from build123d import *

# Parameters (mm, degrees)
F1_DEPTH  = 1120.775
F3_DEPTH  = 53.34
F6_DEPTH  = 565.15
F8_DEPTH  = 55.5625
F10_DEPTH = 45.155127
F12_DEPTH = 25.4
F14_DEPTH = 25.4
F16_DEPTH = 55.5625
F18_DEPTH = 49.193727
F20_DEPTH = 25.4
F22_DEPTH = 113.792
F24_DEPTH = 25.4
F26_DEPTH = 25.4
F28_DEPTH = 25.4
F30_DEPTH = 254
F32_DEPTH = 63.5
F34_DEPTH = 25.4
F36_DEPTH = 25.4
F38_DEPTH = 25.4
F40_DEPTH = 25.4
F41_W     = 53.975
F41_H     = 53.975
F42_DEPTH = 1239.52
F43_R     = 10.31875
F44_DEPTH = 89.662
F45_R     = 10.31875
F46_DEPTH = 179.832


with BuildPart() as f1:
    # F0 (on Front) → F1 (new body)
    with BuildSketch(Plane.XZ):
        Polygon((30.1625, 30.1625), (26.9875, 30.1625), (-26.9875, 30.1625), (-30.1625, 30.1625), (-30.1625, 26.9875), (-30.1625, -26.9875), (-30.1625, -30.1625), (-26.9875, -30.1625), (26.9875, -30.1625), (30.1625, -30.1625), (30.1625, -26.9875), (30.1625, 26.9875), align=None)
        Polygon((-23.8125, 26.9875), (23.8125, 26.9875), (26.9875, 26.9875), (26.9875, 23.8125), (26.9875, -23.8125), (26.9875, -26.9875), (23.8125, -26.9875), (-23.8125, -26.9875), (-26.9875, -26.9875), (-26.9875, -23.8125), (-26.9875, 23.8125), (-26.9875, 26.9875), align=None, mode=Mode.SUBTRACT)
    extrude(amount=-F1_DEPTH)

    # F2 (on Right) → F3 (cut, symmetric)
    with BuildSketch(Plane.YZ):
        Polygon((569.9125, 80.052234), (569.9125, 0), (569.9125, -86.322285), (989.0125, -86.322285), (989.0125, 80.052234), align=None)
    extrude(amount=F3_DEPTH, both=True, mode=Mode.SUBTRACT)



with BuildPart() as f6:
    # F5 (on offset) → F6 (new body)
    with BuildSketch(Plane.XZ.offset(-468.3125)):
        Polygon((-20.5486, 35.0139), (-20.5486, 30.2514), (30.2514, 30.2514), (30.2514, -19.031227), (35.0139, -19.031227), (35.0139, 35.0139), align=None)
        Polygon((-30.2514, 19.031227), (-35.0139, 19.031227), (-35.0139, -35.0139), (20.5486, -35.0139), (20.5486, -30.2514), (-30.2514, -30.2514), align=None)
    extrude(amount=-F6_DEPTH)


with BuildPart() as f1_1:
    add(f1.part)

    add(f6.part)  # F8 merges F6
    # F7 (on face) → F8 (join, through all)
    with BuildSketch(Plane(origin=(-20.5486, 0, 0), x_dir=(0, -1, 0), z_dir=(-1, 0, 0))):
        Polygon((-1033.4625, 30.2514), (-1033.4625, 35.0139), (-1042.3525, 26.1239), (-1033.4625, 26.1239), align=None)
        Polygon((-459.4225, 26.1239), (-468.3125, 35.0139), (-468.3125, 30.2514), (-468.3125, 26.1239), align=None)
    extrude(amount=-F8_DEPTH)

    # F9 (on face) → F10 (join, through all)
    with BuildSketch(Plane(origin=(0, 0, -19.031227), x_dir=(1, 0, 0), z_dir=(0, 0, -1))):
        Polygon((30.2514, -468.3125), (35.0139, -468.3125), (26.1239, -459.4225), (26.1239, -468.3125), align=None)
        Polygon((26.1239, -1042.3525), (35.0139, -1033.4625), (30.2514, -1033.4625), (26.1239, -1033.4625), align=None)
    extrude(amount=-F10_DEPTH)

    # F11 (on face) → F12 (cut)
    with BuildSketch(Plane(origin=(0, 0, 26.1239), x_dir=(1, 0, 0), z_dir=(0, 0, -1))):
        Polygon((35.0139, -459.4225), (30.1625, -459.4225), (30.1625, -463.4611), (35.0139, -468.3125), align=None)
    extrude(amount=-F12_DEPTH, mode=Mode.SUBTRACT)

    # F13 (on face) → F14 (cut)
    with BuildSketch(Plane(origin=(0, 0, 26.1239), x_dir=(1, 0, 0), z_dir=(0, 0, -1))):
        Polygon((35.0139, -1042.3525), (35.0139, -1033.4625), (30.1625, -1038.3139), (30.1625, -1042.3525), align=None)
    extrude(amount=-F14_DEPTH, mode=Mode.SUBTRACT)

    # F15 (on face) → F16 (join, through all)
    with BuildSketch(Plane.YZ.offset(20.5486)):
        Polygon((459.4225, -26.1239), (468.3125, -35.0139), (468.3125, -26.1239), align=None)
        Polygon((1033.4625, -26.1239), (1033.4625, -35.0139), (1042.3525, -26.1239), align=None)
    extrude(amount=-F16_DEPTH)

    # F17 (on face) → F18 (join, through all)
    with BuildSketch(Plane.XY.offset(19.031227)):
        Polygon((-26.1239, 468.3125), (-35.0139, 468.3125), (-26.1239, 459.4225), align=None)
        Polygon((-26.1239, 1042.3525), (-35.0139, 1033.4625), (-26.1239, 1033.4625), align=None)
    extrude(amount=-F18_DEPTH)

    # F19 (on face) → F20 (cut)
    with BuildSketch(Plane.XY.offset(-26.1239)):
        Polygon((-35.0139, 1033.4625), (-30.1625, 1038.3139), (-30.1625, 1042.3525), (-35.0139, 1042.3525), align=None)
    extrude(amount=-F20_DEPTH, mode=Mode.SUBTRACT)

    # F21 (on face) → F22 (join)
    with BuildSketch(Plane(origin=(0, 569.9125, 0), x_dir=(-1, 0, 0), z_dir=(0, 1, 0))):
        Polygon((29.4386, 26.1239), (20.5486, 35.0139), (20.5486, 26.1239), (26.1239, 26.1239), (26.1239, 27.921227), (27.921227, 26.1239), align=None)
        Polygon((27.921227, 26.1239), (26.1239, 26.1239), (26.1239, 19.031227), (35.0139, 19.031227), align=None)
        Polygon((-26.1239, -26.1239), (-26.1239, -19.031227), (-35.0139, -19.031227), (-27.921227, -26.1239), align=None)
        Polygon((-20.5486, -26.1239), (-26.1239, -26.1239), (-26.1239, -27.921227), (-27.921227, -26.1239), (-29.4386, -26.1239), (-20.5486, -35.0139), align=None)
    extrude(amount=-F22_DEPTH)

    # F23 (on face) → F24 (cut)
    with BuildSketch(Plane(origin=(20.5486, 0, 0), x_dir=(0, -1, 0), z_dir=(-1, 0, 0))):
        Polygon((-468.3125, -35.0139), (-456.1205, -35.0139), (-456.1205, -30.1625), (-463.4611, -30.1625), align=None)
    extrude(amount=-F24_DEPTH, mode=Mode.SUBTRACT)

    # F25 (on face) → F26 (cut)
    with BuildSketch(Plane.XY.offset(-19.031227)):
        Polygon((35.0139, 468.3125), (30.1625, 463.4611), (30.1625, 456.1205), (35.0139, 456.1205), align=None)
    extrude(amount=-F26_DEPTH, mode=Mode.SUBTRACT)

    # F27 (on face) → F28 (cut)
    with BuildSketch(Plane.YZ.offset(-20.5486)):
        Polygon((456.1205, 35.0139), (456.1205, 30.1625), (463.4611, 30.1625), (468.3125, 35.0139), align=None)
    extrude(amount=-F28_DEPTH, mode=Mode.SUBTRACT)

    # F29 (on face) → F30 (cut, symmetric)
    with BuildSketch(Plane(origin=(0, 0, 19.031227), x_dir=(1, 0, 0), z_dir=(0, 0, -1))):
        Polygon((-35.0139, -468.3125), (-30.1625, -463.4611), (-30.1625, -456.1205), (-35.0139, -456.1205), align=None)
    extrude(amount=F30_DEPTH, both=True, mode=Mode.SUBTRACT)

    # F31 (on face) → F32 (join)
    with BuildSketch(Plane.XZ.offset(-989.0125)):
        Polygon((-35.0139, 19.031227), (-26.1239, 19.031227), (-26.1239, 26.1239), (-27.921227, 26.1239), align=None)
        Polygon((-26.1239, 27.921227), (-26.1239, 26.1239), (-20.5486, 26.1239), (-20.5486, 35.0139), (-29.4386, 26.1239), (-27.921227, 26.1239), align=None)
        Polygon((20.5486, -26.1239), (20.5486, -35.0139), (29.4386, -26.1239), (27.921227, -26.1239), (26.1239, -27.921227), (26.1239, -26.1239), align=None)
        Polygon((26.1239, -19.031227), (26.1239, -26.1239), (27.921227, -26.1239), (35.0139, -19.031227), align=None)
    extrude(amount=-F32_DEPTH)

    # F33 (on face) → F34 (cut)
    with BuildSketch(Plane(origin=(20.5486, 0, 0), x_dir=(0, -1, 0), z_dir=(-1, 0, 0))):
        Polygon((-1052.5125, -35.0139), (-1033.4625, -35.0139), (-1038.3139, -30.1625), (-1052.5125, -30.1625), align=None)
    extrude(amount=-F34_DEPTH, mode=Mode.SUBTRACT)

    # F35 (on face) → F36 (cut)
    with BuildSketch(Plane(origin=(0, 0, 19.031227), x_dir=(1, 0, 0), z_dir=(0, 0, -1))):
        Polygon((-30.1625, -1038.3139), (-35.0139, -1033.4625), (-35.0139, -1052.5125), (-30.1625, -1052.5125), align=None)
    extrude(amount=-F36_DEPTH, mode=Mode.SUBTRACT)

    # F37 (on face) → F38 (cut)
    with BuildSketch(Plane.YZ.offset(-20.5486)):
        Polygon((1052.5125, 35.0139), (1033.4625, 35.0139), (1038.3139, 30.1625), (1052.5125, 30.1625), align=None)
    extrude(amount=-F38_DEPTH, mode=Mode.SUBTRACT)

    # F39 (on face) → F40 (cut)
    with BuildSketch(Plane.XY.offset(-19.031227)):
        Polygon((30.1625, 1052.5125), (30.1625, 1038.3139), (35.0139, 1033.4625), (35.0139, 1052.5125), align=None)
    extrude(amount=-F40_DEPTH, mode=Mode.SUBTRACT)

    # F41 (on face) → F42 (cut)
    with BuildSketch(Plane.XZ):
        Rectangle(F41_W, F41_H)
    extrude(amount=-F42_DEPTH, mode=Mode.SUBTRACT)

    # F43 (on face) → F44 (cut)
    with BuildSketch(Plane(origin=(-30.1625, 0, 0), x_dir=(0, -1, 0), z_dir=(-1, 0, 0))):
        with Locations((-1059.65625, 11.1125)):
            Circle(F43_R)
    extrude(amount=-F44_DEPTH, mode=Mode.SUBTRACT)

    # F45 (on face) → F46 (cut)
    with BuildSketch(Plane(origin=(-30.1625, 0, 0), x_dir=(0, -1, 0), z_dir=(-1, 0, 0))):
        with Locations((-111.125, 0)):
            Circle(F45_R)
    extrude(amount=-F46_DEPTH, mode=Mode.SUBTRACT)


solid = f1_1.part
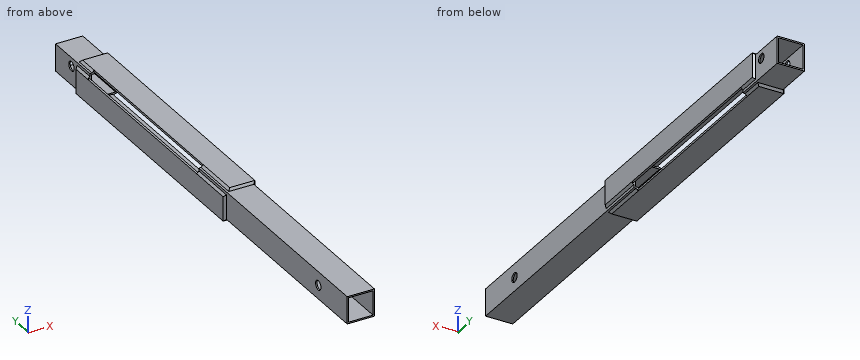
For this review, take the finished solid that the model builds, in its own axes (mm). Round coordinates to 2 decimals unless told otherwise and drop trailing zeros. Write each loop counter-clockwise with the first axis right and the second up, starting at its lowest first coordinate (ties: lowest second). Pieces come first, ordered by that corner, then holes. Notation, with made-up numbers: M 81.5,12 L 98.5,12 A21 ccw 98.5,43 Z; hole C 57,35.5 d5. An arc over 180 degrees is marked long. Write item = value, one per line. Start each with the question number.
(1) We need section B-B (y = 208). Give the boundary of the cut face in (x, z).
(2) We need section C-C (y = 492.5). Give the boundary of the cut face in (x, z), then the cut area to 3 significant figures.
(3) For line 1 along Z through (x, y) = (26, 193); line 2 along Z through (x, y) = (6, 805), list the stretches that pass through material, from the lowest coordinate up.
(4) Clearance check with flat-ended pins moving along their axes: pin 1 Ø3 at (y, z) = (261.5, 7) entering from -X; pin 2 Ø8 at (x, z) = (21.5, 0) entering from +Y; pin 3 Ø3 at (y, z) = (973, -21.5) entering from +X; pin 4 Ø5 at (y, z) = (787, -33.5) entering from +X. State where each tip first meets the part, or that it passes through.
Results found:
q1.outline = M -30.16,-30.16 L 30.16,-30.16 L 30.16,30.16 L -30.16,30.16 Z; hole M -26.99,-26.99 L 26.99,-26.99 L 26.99,26.99 L -26.99,26.99 Z
q2.outline = M -35.01,-35.01 L 20.55,-35.01 L 25.4,-30.16 L 30.16,-30.16 L 30.16,-23.88 L 35.01,-19.03 L 35.01,35.01 L -20.55,35.01 L -25.4,30.16 L -30.16,30.16 L -30.16,23.88 L -35.01,19.03 Z; hole M -30.25,-30.25 L 20.55,-30.25 L 20.55,-30.16 L -30.16,-30.16 L -30.16,19.03 L -30.25,19.03 Z; hole M -26.99,-26.99 L 26.99,-26.99 L 26.99,26.99 L -26.99,26.99 Z; hole M -20.55,30.16 L 30.16,30.16 L 30.16,-19.03 L 30.25,-19.03 L 30.25,30.25 L -20.55,30.25 Z
q2.area = 1,770 mm²
q3.line_1 = -30.16 to -26.99, 26.99 to 30.16
q3.line_2 = -35.01 to -30.25, 30.25 to 35.01
q4.pin_1 = -30.16
q4.pin_2 = through
q4.pin_3 = -30.25
q4.pin_4 = 20.55
